from build123d import *

# Parameters (mm, degrees)
SKETCH1_R                 = 4
BOSS_EXTRUDE1_DEPTH       = 21
SKETCH2_W                 = 19
SKETCH2_H                 = 11
CUT_EXTRUDE1_DEPTH        = 20
SKETCH3_R                 = 8.5
CUT_EXTRUDE2_DEPTH        = 12
M2X0_4_TAPPED_HOLE1_D     = 1.6
M2X0_4_TAPPED_HOLE1_DEPTH = 8
M2X0_4_TAPPED_HOLE1_TIP   = 0.480688495
FILLET2_R                 = 3
CHAMFER1_SIZE             = 3
FILLET3_R                 = 2


with BuildPart() as part:
    # Sketch1 → Boss-Extrude1 (new body)
    with BuildSketch(Plane.XY):
        with BuildLine():
            Line((0, 0), (0, 20))
            Line((0, 20), (23, 20))
            ThreePointArc((23, 20), (33, 10), (23, 0))
            Line((23, 0), (0, 0))
        make_face()
        with Locations(Location((25, 10, 0), (0, 0, 180))):
            Circle(SKETCH1_R, mode=Mode.SUBTRACT)
    extrude(amount=BOSS_EXTRUDE1_DEPTH)

    # Sketch2 → Cut-Extrude1 (cut)
    with BuildSketch(Plane(origin=(0, 20, 0), x_dir=(1, 0, 0), z_dir=(0, 1, 0))):
        with Locations((23.5, -10.5)):
            Rectangle(SKETCH2_W, SKETCH2_H)
    extrude(amount=-CUT_EXTRUDE1_DEPTH, mode=Mode.SUBTRACT)

    # Sketch3 → Cut-Extrude2 (cut)
    with BuildSketch(Plane.ZY):
        with Locations(Location((10.5, 10, 0), (0, 0, 270))):
            Circle(SKETCH3_R)
    extrude(amount=-CUT_EXTRUDE2_DEPTH, mode=Mode.SUBTRACT)

    # M2x0.4 Tapped Hole1
    with Locations(Plane.ZY):
        with Locations((2, 17.5), (19, 17.5), (19, 2.5), (2, 2.5)):
            Hole(M2X0_4_TAPPED_HOLE1_D / 2, depth=M2X0_4_TAPPED_HOLE1_DEPTH)
            with Locations((0, 0, -(M2X0_4_TAPPED_HOLE1_DEPTH + M2X0_4_TAPPED_HOLE1_TIP / 2))):  # 118° drill point
                Cone(0, M2X0_4_TAPPED_HOLE1_D / 2, M2X0_4_TAPPED_HOLE1_TIP, mode=Mode.SUBTRACT)

    # Fillet2
    fillet2_edges = [part.edges().sort_by_distance(p)[0] for p in [
        (11.5, 20, 21),
        (11.5, 0, 21),
        (11.5, 20, 0),
        (33, 10, 0),
        (11.5, 0, 0),
        (33, 10, 21),
    ]]
    fillet(fillet2_edges, radius=FILLET2_R)

    # Chamfer1
    chamfer1_edges = [part.edges().sort_by_distance(p)[0] for p in [
        (14, 0, 10.5),
        (14, 20, 10.5),
    ]]
    chamfer(chamfer1_edges, length=CHAMFER1_SIZE)

    # Fillet3
    fillet3_edges = [part.edges().sort_by_distance(p)[0] for p in [
        (14, 17, 10.5),
        (14, 3, 10.5),
        (11, 0, 10.5),
        (11, 20, 10.5),
    ]]
    fillet(fillet3_edges, radius=FILLET3_R)


solid = part.part
Part model, mm, in its own coordinate system. A direction names the side the tool comes from. Coordinates: 2 decimals unless noted, no trailing zeros. Order: outer loops, then holes, each group sorted by start corner. A loop starts at its lowest first (then second) coordinate and runs counter-clockwise, first axis right, second up.
(1) Probe L1, parallel to Z at x = 21, y = 5.25; L2, parallel to Z at x = 3.5, y = 2.5; L3, parallel to Z at x = 3.5, y = 10. List the from-to ranges inside material, lowest first.
Check sheet entries:
L1: z = 0 to 5, 16 to 21
L2: z = 0.04 to 1.2, 2.8 to 6.5, 14.5 to 18.2, 19.8 to 20.96
L3: z = 0 to 2, 19 to 21
(2) Slice it at B-B, the plane x = 3. Write the cut outline in (y, z).
Check sheet entries:
outline: (0, 3) arc R3 ccw to (3, 0) - (17, 0) arc R3 ccw to (20, 3) - (20, 18) arc R3 ccw to (17, 21) - (3, 21) arc R3 ccw to (0, 18) - close; hole circle Ø17 at (10, 10.5); hole circle Ø1.6 at (2.5, 2); hole circle Ø1.6 at (2.5, 19); hole circle Ø1.6 at (17.5, 2); hole circle Ø1.6 at (17.5, 19)
(3) Tool access for faces 1 (the face through (7, 0, 10)), 2 (the face through (5.916, 16.745, 5.328)), 3 (the face through (13, 2, 11)): list every direction of +Z, -Z, +X, -X, +Y, -Y with a clear straight run to the whole face (end or side of a thin tool).
Check sheet entries:
face 1: +Z, -Z, +X, -X, -Y
face 2: -X
face 3: +X, -Y
(4) Pin check, flat tips, straight feed: pin 1 Ø1 at (y, z) = (2.5, 2) entering from -X; pin 2 Ø12 at (y, z) = (10, 11.5) entering from +X; pin 3 Ø1.4 at (y, z) = (2.5, 19) entering from +X. Stop position of each tip, or through.
Check sheet entries:
pin 1: stops at x = 8.18
pin 2: stops at x = 33
pin 3: stops at x = 30.16
(5) Pull direction Y, two halves, no side cores. Call faces 4 (the face through (8.4, 2.38, 2.06)), 5 (the face through (13, 18, 11)), 6 (the face through (28.2, 12.4, 2.5)), 7 (the face through (14, 10, 11)): pulls with the +Y half, pulls with the -Y half, needs draft (parallel to the pull), parting line crosses it, or undercut.
Check sheet entries:
face 4: undercut
face 5: pulls with the +Y half
face 6: undercut
face 7: needs draft
(6) Slice it at A-A, the plane x = 16. Write the cut outline in (y, z), and give its area (3 significant figures).
Check sheet entries:
outline: (0, 3) arc R3 ccw to (3, 0) - (17, 0) arc R3 ccw to (20, 3) - (20, 5) - (0, 5) - close; (0, 16) - (20, 16) - (20, 18) arc R3 ccw to (17, 21) - (3, 21) arc R3 ccw to (0, 18) - close
area: 192 mm2
(7) Slice it at D-D, the plane z = 4. Write the cut outline in (x, y).
Check sheet entries:
outline: (0, 0) - (23, 0) arc R10 ccw to (23, 20) - (0, 20) - (0, 15.48) - (12, 15.48) - (12, 4.52) - (0, 4.52) - close; hole circle Ø8 at (25, 10)
(8) Slice it at C-C, the plane z = 10.5. Write the cut outline in (x, y).
Check sheet entries:
outline: (0, 0) - (10.17, 0) arc R2 ccw to (11.59, 0.59) - (13.41, 2.41) arc R2 ccw to (14, 3.83) - (14, 16.17) arc R2 ccw to (13.41, 17.59) - (11.59, 19.41) arc R2 ccw to (10.17, 20) - (0, 20) - (0, 18.5) - (12, 18.5) - (12, 1.5) - (0, 1.5) - close
